Build history of the part. All positions in model axes, mm. Face numbers are marked on the shaded views. Round coordinates to 2 decimals unless told otherwise and drop trailing zeros. Order: outer loops, then holes, each group sorted by start corner. A loop starts at its lowest first (then second) coordinate and runs counter-clockwise, first axis right, second up. Notation, with made-up numbers: (-15, 31.25) -> (38, 31.25) arc R29 ccw to (38, 53.25) -> close; hole circle Ø7 at (13, 1). An arc over 180 degrees is marked (long way). Write item = value, one per line.
Autodesk Inventor part; units mm, degrees
ref_plane "YZ Plane" through (0, 0, 0) normal (1, 0, 0) x (0, 1, 0)
ref_plane "XZ Plane" through (0, 0, 0) normal (0, 1, 0) x (-1, 0, 0)
ref_plane "XY Plane" through (0, 0, 0) normal (0, 0, 1) x (1, 0, 0)
sketch "Sketch1" plane through (0, 0, 0) normal (0, 0, 1) x (1, 0, 0)
  line L0 (0, 0) -> (60, 0)
  line L1 (60, 0) -> (60, 10)
  line L2 (60, 10) -> (0, 10)
  line L3 (0, 10) -> (0, 0)
  dimension "d0" = 60
  dimension "d1" = 10
extrude "Extrusion1" add sketch "Sketch1" along normal blind 2
fillet "Fillet1" radius 5 4 edges at (0, 10, 1) (0, 0, 1) (60, 10, 1) (60, 0, 1)
sketch "Sketch2" plane through (0, 0, 2) normal (0, 0, 1) x (1, 0, 0)
  arc A0 (5, 10) -> (5, 0) centre (5, 5) ccw
  circle A1 centre (5, 5) radius 1.5
  arc A2 (55, 0) -> (55, 10) centre (55, 5) ccw
  circle A3 centre (55, 5) radius 1.5
  line L0 (55, 10) -> (5, 10)
  line L1 (30, 10) -> (30, 5)
  line L2 (30, 5) -> (35, 5)
  circle A4 centre (35, 5) radius 1.5
  point P0 (0, 0)
  dimension "d5" = 3
  dimension "d6" = 3
  dimension "d9" = 5
  dimension "d10" = 3
extrude "Extrusion2" cut sketch "Sketch2" against normal blind 2
properties part number "Side Support 2"
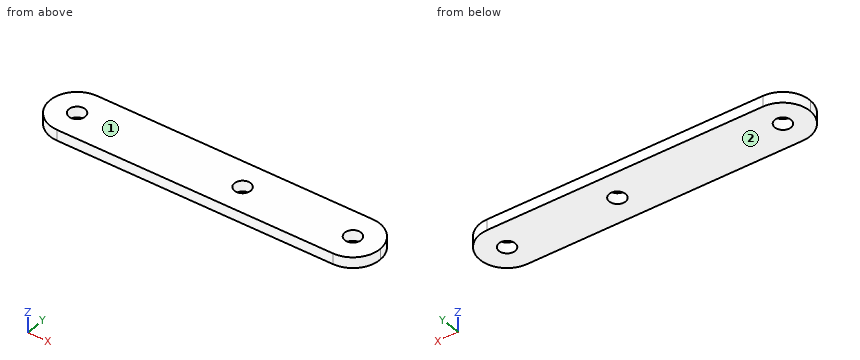
Q1. Cut at C-C, the plane y = 5.5. List the corners of the cut face in (x, z).
Check values:
outline = (0.03, 0) -> (3.59, 0) -> (3.59, 2) -> (0.03, 2) -> close; (6.41, 0) -> (33.59, 0) -> (33.59, 2) -> (6.41, 2) -> close; (36.41, 0) -> (53.59, 0) -> (53.59, 2) -> (36.41, 2) -> close; (56.41, 0) -> (59.97, 0) -> (59.97, 2) -> (56.41, 2) -> close
Q2. Mould opens along Z. For the marked faces 1 and 2 say: released by +Z, released by -Z, zero draft, split by the parting line, or undercut.
Check values:
face_1 = released by +Z
face_2 = released by -Z
Q3. Cut at B-B, the plane z = 0.8. Give the number of separate pieces and of enclosed holes in the cut face, and give its area (3 significant figures).
Check values:
separate_pieces = 1
enclosed_holes = 3
area = 557 mm²
Q4. Cut at A-A, the plane x = 35. List the corners of the cut face in (y, z), and give its area (3 significant figures).
Check values:
outline = (0, 0) -> (3.5, 0) -> (3.5, 2) -> (0, 2) -> close; (6.5, 0) -> (10, 0) -> (10, 2) -> (6.5, 2) -> close
area = 14.0 mm²
Q5. Cut at D-D, the plane x = 54.5. List the corners of the cut face in (y, z), and give its area (3 significant figures).
Check values:
outline = (0, 0) -> (3.59, 0) -> (3.59, 2) -> (0, 2) -> close; (6.41, 0) -> (10, 0) -> (10, 2) -> (6.41, 2) -> close
area = 14.3 mm²
Q6. Probe probe 1 along Y at (x, z) = (35, 0.85); probe 2 along X at (y, z) = (5.75, 0.3); probe 3 along X at (y, z) = (5.25, 0.55). List the from-to ranges inside material, lowest first.
Check values:
probe_1 = 0 to 3.5, 6.5 to 10
probe_2 = 0.06 to 3.7, 6.3 to 33.7, 36.3 to 53.7, 56.3 to 59.94
probe_3 = 0.01 to 3.52, 6.48 to 33.52, 36.48 to 53.52, 56.48 to 59.99
